Read the model definition and answer for the solid it produces. Units are mm, in the model's axes. Coordinates: 2 decimals unless noted, no trailing zeros. Write each loop counter-clockwise with the first axis right and the second up, starting at its lowest first coordinate (ties: lowest second). Pieces come first, ordered by that corner, then holes.
(1) Section A-A on y = 39.5 is taken. Write down the section's boundary in (x, z).
(2) Section D-D on y = 5 is taken. Write down the section's boundary in (x, z).
(3) Section B-B on x = 0 is taken. Write down the section's boundary in (y, z), then the cut area to 3 significant figures.
(4) Section C-C on z = 0.5 is taken. Write down the section's boundary in (x, y), then the cut area to 3 significant figures.
(5) The mould has two halves that part along X. Classify faces 1 (the flat face through (0, 1, 2)), 2 (the cylindrical face through (-0.521, 43.466, 1.014)), 3 (the flat face through (9, -49, 1)), 4 (the cylindrical face through (-1.5, 5.07, 1.01)): +X half, -X half, draft (parallel to the pull), parting line (faces both ways), or undercut.
(6) Given pin 1 (6.5 mm diameter, centred on x = 0, y = 39.5, fed in from +Z); pin 2 (4 mm diameter, centred on x = 0, y = 5, fed in from -Z), each flat-ended and moving along its own axis, determine where each tip first touches the part or whether it passes through.
(7) Find the intervals of material crossed by probe 1 along Y at (x, z) = (0, 1.45); probe 2 along Y at (x, z) = (-1, 1.9); probe 3 along X at (y, z) = (37.5, 1.2), in increasing order.
from build123d import *

# Parameters (mm, degrees)
SKETCH1_W           = 20
SKETCH1_H           = 100
BOSS_EXTRUDE1_DEPTH = 2
CUT_EXTRUDE1_REACH  = 53.029
SKETCH2_R           = 4
SKETCH2_R_2         = 1.5
SKETCH2_R_3         = 3.5
CHAMFER1_SIZE       = 2


with BuildPart() as part:
    # Sketch1 → Boss-Extrude1 (new body)
    with BuildSketch(Plane.XY):
        Rectangle(SKETCH1_W, SKETCH1_H)
    extrude(amount=BOSS_EXTRUDE1_DEPTH)

    # Sketch2 → Cut-Extrude1 (cut, up to next)
    with BuildSketch(Plane.XY.offset(2), mode=Mode.PRIVATE) as cut_extrude1_sk1:
        with Locations((0, 39.5)):
            Circle(SKETCH2_R)
    cut_extrude1_tool1 = extrude(cut_extrude1_sk1.sketch, amount=-CUT_EXTRUDE1_REACH, mode=Mode.PRIVATE) & part.part
    # Sketch2 → Cut-Extrude1 (cut, up to next)
    with BuildSketch(Plane.XY.offset(2), mode=Mode.PRIVATE) as cut_extrude1_sk2:
        with Locations((0, 5)):
            Circle(SKETCH2_R_2)
    cut_extrude1_tool2 = extrude(cut_extrude1_sk2.sketch, amount=-CUT_EXTRUDE1_REACH, mode=Mode.PRIVATE) & part.part
    # Sketch2 → Cut-Extrude1 (cut, up to next)
    with BuildSketch(Plane.XY.offset(2), mode=Mode.PRIVATE) as cut_extrude1_sk3:
        with Locations((0, -30)):
            Circle(SKETCH2_R_3)
    cut_extrude1_tool3 = extrude(cut_extrude1_sk3.sketch, amount=-CUT_EXTRUDE1_REACH, mode=Mode.PRIVATE) & part.part
    add(cut_extrude1_tool1.solids().sort_by_distance((0, 39.5, 2))[0], mode=Mode.SUBTRACT)
    add(cut_extrude1_tool2.solids().sort_by_distance((0, 5, 2))[0], mode=Mode.SUBTRACT)
    add(cut_extrude1_tool3.solids().sort_by_distance((0, -30, 2))[0], mode=Mode.SUBTRACT)

    # Chamfer1
    chamfer1_edges = [part.edges().sort_by_distance(p)[0] for p in [
        (10, -50, 1),
        (-10, -50, 1),
        (-10, 50, 1),
        (10, 50, 1),
    ]]
    chamfer(chamfer1_edges, length=CHAMFER1_SIZE)


solid = part.part
Response:
1. outline: (-10, 0) - (-4, 0) - (-4, 2) - (-10, 2) - close; (4, 0) - (10, 0) - (10, 2) - (4, 2) - close
2. outline: (-10, 0) - (-1.5, 0) - (-1.5, 2) - (-10, 2) - close; (1.5, 0) - (10, 0) - (10, 2) - (1.5, 2) - close
3. outline: (-50, 0) - (-33.5, 0) - (-33.5, 2) - (-50, 2) - close; (-26.5, 0) - (3.5, 0) - (3.5, 2) - (-26.5, 2) - close; (6.5, 0) - (35.5, 0) - (35.5, 2) - (6.5, 2) - close; (43.5, 0) - (50, 0) - (50, 2) - (43.5, 2) - close
3. area: 164 mm2
4. outline: (-10, -48) - (-8, -50) - (8, -50) - (10, -48) - (10, 48) - (8, 50) - (-8, 50) - (-10, 48) - close; hole circle Ø8 at (0, 39.5); hole circle Ø7 at (0, -30); hole circle Ø3 at (0, 5)
4. area: 1,900 mm2
5. face 1: draft
5. face 2: undercut
5. face 3: +X half
5. face 4: undercut
6. pin 1: passes through
6. pin 2: stops at z = 0
7. probe 1: y = -50 to -33.5, -26.5 to 3.5, 6.5 to 35.5, 43.5 to 50
7. probe 2: y = -50 to -33.35, -26.65 to 3.88, 6.12 to 35.63, 43.37 to 50
7. probe 3: x = -10 to -3.46, 3.46 to 10
